Part model, mm, in its own coordinate system. Coordinates: 2 decimals unless noted, no trailing zeros. Write each loop counter-clockwise with the first axis right and the second up, starting at its lowest first coordinate (ties: lowest second). Pieces come first, ordered by that corner, then holes. Notation, with made-up numbers: M 24.25,-27.5 L 62.25,-27.5 A23 ccw 62.25,-10.5 Z; hole C -4,-24 d2. An arc over 180 degrees is marked long. Use a Markdown table: item, result. Add a question column.
Q1. Slice it at D-D on y = -2.1. Count the separate pieces of the cut face and the enclosed holes in it, then the cut area to 3 significant figures.
Q2. Pin check, flat tip, straight feed: pin 1 Ø2.5 at (x, z) = (0, -10.1) entering from +Y. Stop position of the tip, or through.
Q3. Slice it at A-A on x = 0. Write the cut outline in (y, z) (3 decimals), then the cut area to 3 significant figures.
Q4. Slice it at C-C on x = 20. Write the cut outline in (y, z) (3 decimals), then the cut area to 3 significant figures.
Q5. Wall check: L1, parallel to X at y = -0.95, z = 160; L2, parallel to Z at x = 19.5, y = -1.6; L3, parallel to Z at x = -10, y = -2.1. Give the ranges that are in metal, low to high. Write a range as from..to.
Q6. Slice it at B-B on z = 160. Write the cut outline in (x, y) (3 decimals), then the cut area to 4 significant figures.
from build123d import *

# Parameters (mm, degrees)
BASE_FLANGE1_DEPTH = 3.125
SKETCH4_R          = 1.6
CUT_EXTRUDE1_DEPTH = 167.912448981
SKETCH6_R          = 1.6
CUT_EXTRUDE3_DEPTH = 167.912448981


# Sheet-metal steps are written as plain solids
with BuildPart() as part:
    # Sketch1 → Base-Flange1 (new body)
    with BuildSketch(Plane(origin=(0, 0, 0), x_dir=(1, 0, 0), z_dir=(0, 1, 0))):
        with BuildLine():
            Line((-25, 0), (-25, -140))
            ThreePointArc((-25, -140), (0, -165), (25, -140))
            Line((25, -140), (25, 0))
            ThreePointArc((25, 0), (0, 25), (-25, 0))
        make_face()
    extrude(amount=-BASE_FLANGE1_DEPTH)

    # Sketch4 → Cut-Extrude1 (cut, through all)
    with BuildSketch(Plane.XZ.offset(3.125)):
        with Locations(Location((0, -10.098593171, 0), (0, 0, 270))):
            Circle(SKETCH4_R)
        with Locations(Location((10.098593171, 0, 0), (0, 0, 270))):
            Circle(SKETCH4_R)
        with Locations(Location((-10.098593171, 0, 0), (0, 0, 270))):
            Circle(SKETCH4_R)
        with Locations(Location((0, 10.098593171, 0), (0, 0, 270))):
            Circle(SKETCH4_R)
    extrude(amount=-CUT_EXTRUDE1_DEPTH, mode=Mode.SUBTRACT)

    # Sketch6 → Cut-Extrude3 (cut, through all)
    with BuildSketch(Plane(origin=(0, 0, 0), x_dir=(1, 0, 0), z_dir=(0, 1, 0))):
        with Locations(Location((0, -120, 0), (0, 0, 270))):
            Circle(SKETCH6_R)
        with Locations(Location((-20, -140, 0), (0, 0, 270))):
            Circle(SKETCH6_R)
        with Locations(Location((0, -160, 0), (0, 0, 270))):
            Circle(SKETCH6_R)
        with Locations(Location((20, -140, 0), (0, 0, 270))):
            Circle(SKETCH6_R)
    extrude(amount=-CUT_EXTRUDE3_DEPTH, mode=Mode.SUBTRACT)


solid = part.part
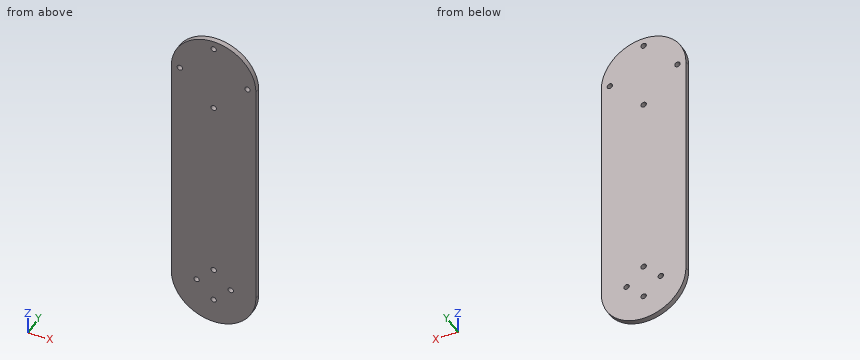
Recorded:
| question | item | result |
|---|---|---|
| 1 | separate pieces | 1 |
| 1 | enclosed holes | 8 |
| 1 | area | 8,900 mm² |
| 2 | pin 1 | through |
| 3 | outline | M -3.125,-25 L 0,-25 L 0,-11.699 L -3.125,-11.699 Z; M -3.125,-8.499 L 0,-8.499 L 0,8.499 L -3.125,8.499 Z; M -3.125,11.699 L 0,11.699 L 0,118.4 L -3.125,118.4 Z; M -3.125,121.6 L 0,121.6 L 0,158.4 L -3.125,158.4 Z; M -3.125,161.6 L 0,161.6 L 0,165 L -3.125,165 Z |
| 3 | area | 554 mm² |
| 4 | outline | M -3.125,-15 L 0,-15 L 0,138.4 L -3.125,138.4 Z; M -3.125,141.6 L 0,141.6 L 0,155 L -3.125,155 Z |
| 4 | area | 521 mm² |
| 5 | L1 | -15..-1.6, 1.6..15 |
| 5 | L2 | -15.64..138.48, 141.52..155.64 |
| 5 | L3 | -22.91..-1.6, 1.6..162.91 |
| 6 | outline | M -15,-3.125 L -1.6,-3.125 L -1.6,0 L -15,0 Z; M 1.6,-3.125 L 15,-3.125 L 15,0 L 1.6,0 Z |
| 6 | area | 83.75 mm² |
